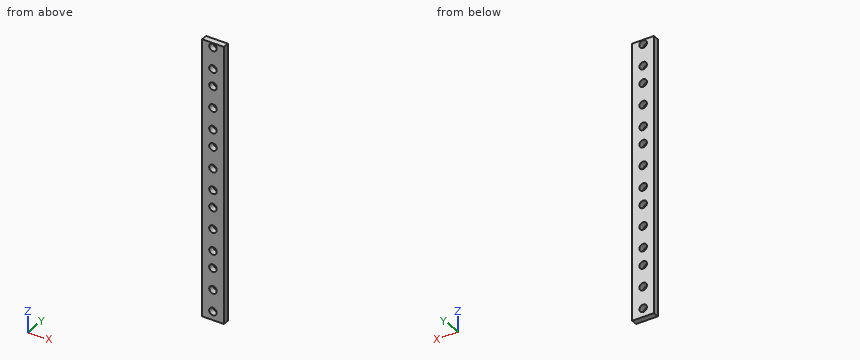
```python
from build123d import *

# Parameters (mm, degrees)
SKETCH_W  = 15.875
SKETCH_H  = 203.2
SKETCH_R  = 2.775
PAD_DEPTH = 4.4


with BuildPart() as part:
    # Sketch → Pad (new body)
    with BuildSketch(Plane.XZ):
        with Locations((7.9375, 101.6)):
            Rectangle(SKETCH_W, SKETCH_H)
        with Locations((7.874, 6.35)):
            Circle(SKETCH_R, mode=Mode.SUBTRACT)
        with Locations((7.874, 22.23)):
            Circle(SKETCH_R, mode=Mode.SUBTRACT)
        with Locations((7.874, 38.11)):
            Circle(SKETCH_R, mode=Mode.SUBTRACT)
        with Locations((7.874, 50.81)):
            Circle(SKETCH_R, mode=Mode.SUBTRACT)
        with Locations((7.874, 66.69)):
            Circle(SKETCH_R, mode=Mode.SUBTRACT)
        with Locations((7.874, 82.57)):
            Circle(SKETCH_R, mode=Mode.SUBTRACT)
        with Locations((7.874, 95.27)):
            Circle(SKETCH_R, mode=Mode.SUBTRACT)
        with Locations((7.874, 111.15)):
            Circle(SKETCH_R, mode=Mode.SUBTRACT)
        with Locations((7.874, 127.03)):
            Circle(SKETCH_R, mode=Mode.SUBTRACT)
        with Locations((7.874, 139.73)):
            Circle(SKETCH_R, mode=Mode.SUBTRACT)
        with Locations((7.874, 155.61)):
            Circle(SKETCH_R, mode=Mode.SUBTRACT)
        with Locations((7.874, 171.49)):
            Circle(SKETCH_R, mode=Mode.SUBTRACT)
        with Locations((7.874, 184.19)):
            Circle(SKETCH_R, mode=Mode.SUBTRACT)
        with Locations((7.874, 200.065)):
            Circle(SKETCH_R, mode=Mode.SUBTRACT)
    extrude(amount=PAD_DEPTH)


solid = part.part
```
Could you check a few things on this model? Use its own coordinates, in mm. Round coordinates to 2 decimals unless told otherwise and drop trailing zeros. Loops run counter-clockwise (first coordinate to the right, second up) from the corner with the lowest first, then second, coordinate; pieces in that order, holes last. Notation, with made-up numbers: (0.5, -23.5) - (13.5, -23.5) arc R18 ccw to (13.5, -6.5) - close; hole circle Ø7 at (87, 28). An arc over 180 degrees is marked (long way). Answer as CSV lines item,"result".
1. I want a section at A-A on z = 82.57. List the corners of the cut face in (x, y) for me (3 decimals), then the cut area to 3 significant figures.
Filled in:
outline,"(0, -4.4) - (5.099, -4.4) - (5.099, 0) - (0, 0) - close; (10.649, -4.4) - (15.875, -4.4) - (15.875, 0) - (10.649, 0) - close"
area,"45.4 mm^2"
2. Please list where these lines run through material, in increasing order: line 1 along X through (y, z) = (-2.8, 184.19) (3 decimals); line 2 along X through (y, z) = (-2.1, 39) (3 decimals). Write a range as [from, to].
Filled in:
line 1,"x = [0, 5.099], [10.649, 15.875]"
line 2,"x = [0, 5.246], [10.502, 15.875]"
3. I want a section at B-B on y = -2.5. Count the separate pieces of the cut face and the enclosed holes in it, then the cut area to 3 significant figures.
Filled in:
separate pieces,"1"
enclosed holes,"14"
area,"2,890 mm^2"
